```python
from build123d import *
from build123d.topology import SkipClean

# Parameters (mm, degrees)
EXTRUDE_1_DEPTH               = 15
CUT_EXTRUDE_1_DEPTH           = 4
SKETCH_3_R                    = 14
CUT_EXTRUDE_2_DEPTH           = 227.475164201
EXTRUDE_4_DEPTH               = 15
SKETCH_11_W                   = 17
SKETCH_11_H                   = 10
SKETCH_14_W                   = 6
SKETCH_14_H                   = 10
CUT_REVOLVE_4_ANGLE           = 60
CUT_REVOLVE_4_OTHER_WAY_ANGLE = 90
SKETCH_16_W                   = 9.609453317
SKETCH_16_H                   = 10
CUT_EXTRUDE_4_DEPTH           = 5
SKETCH_17_W                   = 9.609453317
SKETCH_17_H                   = 10
CUT_EXTRUDE_5_DEPTH           = 5
CUT_EXTRUDE_6_DEPTH           = 7.5
EXTRUDE_START                 = 1.5
EXTRUDE_6_DEPTH               = 1.5
SKETCH_21_R                   = 5
SKETCH_21_R_2                 = 14
EXTRUDE_7_DEPTH               = 1.5
HOLE_WIZARD_M4_1_D            = 3.3
HOLE_WIZARD_M4_1_DEPTH        = 9
HOLE_WIZARD_M4_1_CSINK_D      = 4.05
HOLE_WIZARD_M4_1_CSINK_ANGLE  = 90


with BuildPart() as part:
    # 草图1 → 凸台-拉伸1 (new body)
    with BuildSketch(Plane(origin=(0, 0, 0), x_dir=(1, 0, 0), z_dir=(0, 1, 0))):
        with BuildLine():
            Line((-21, 0), (-21, -215))
            ThreePointArc((-21, -215), (-18.071067812, -222.071067812), (-11, -225))
            Line((-11, -225), (-9.110127779, -225))
            ThreePointArc((-9.110127779, -225), (-2.375625019, -222.392325249), (0.846599179, -215.929294516))
            Line((0.846599179, -215.929294516), (21, 0))
            ThreePointArc((21, 0), (0, 21), (-21, 0))
        make_face()
    extrude(amount=EXTRUDE_1_DEPTH)

    # 草图2 → 切除-拉伸1 (cut)
    with BuildSketch(Plane.XZ):
        with BuildLine():
            Line((-6.487547308, 24.545681698), (-15.16946684, 197.954199749))
            ThreePointArc((-15.16946684, 197.954199749), (-9.006726896, 204.766554422), (-2.194372223, 198.603814478))
            Line((-2.194372223, 198.603814478), (6.487547308, 25.195296427))
            ThreePointArc((6.487547308, 25.195296427), (0.324807364, 18.382941754), (-6.487547308, 24.545681698))
        make_face()
    extrude(amount=-CUT_EXTRUDE_1_DEPTH, mode=Mode.SUBTRACT)

    # 草图3 → 切除-拉伸2 (cut, through all)
    with BuildSketch(Plane(origin=(0, 0, 0), x_dir=(-1, 0, 0), z_dir=(0, -1, 0))):
        with Locations(Location((0, 0, 0), (0, 0, 90))):
            Circle(SKETCH_3_R)
    extrude(amount=-CUT_EXTRUDE_2_DEPTH, mode=Mode.SUBTRACT)

    # 草图7 → 凸台-拉伸4 (add)
    with BuildSketch(Plane(origin=(0, 0, 0), x_dir=(1, 0, 0), z_dir=(0, 1, 0))):
        with BuildLine():
            Line((-10.693069191, 38.039100971), (-19.9158097, 6.66036966))
            ThreePointArc((-19.9158097, 6.66036966), (0, 21), (19.9158097, 6.66036966))
            Line((19.9158097, 6.66036966), (10.693069191, 38.039100971))
            ThreePointArc((10.693069191, 38.039100971), (0, 47.113526612), (-10.693069191, 38.039100971))
        make_face()
    extrude(amount=EXTRUDE_4_DEPTH)

    # 草图11 → 切除-旋转3 (revolve, cut)
    with BuildSketch(Plane(origin=(0, 0, 0), x_dir=(0, 0, -1), z_dir=(1, 0, 0)), mode=Mode.PRIVATE) as cut_revolve_3_sk:
        with Locations((51.539100971, 7.5)):
            Rectangle(SKETCH_11_W, SKETCH_11_H)
    revolve(cut_revolve_3_sk.sketch.rotate(Axis((0, 15, -38.039100971), (0, -1, 0)), 180), axis=Axis((0, 15, -38.039100971), (0, -1, 0)), mode=Mode.SUBTRACT)

    # 草图14 → 切除-旋转4 (revolve, cut)
    with BuildSketch(Plane(origin=(0, 0, 0), x_dir=(0, 0, -1), z_dir=(1, 0, 0))):
        with Locations((19.26034239, 7.5)):
            Rectangle(SKETCH_14_W, SKETCH_14_H)
    revolve(axis=Axis((0, 15, 0), (0, -1, 0)), revolution_arc=CUT_REVOLVE_4_ANGLE, mode=Mode.SUBTRACT)

    # 草图14 → 切除-旋转4 other way (revolve, cut)
    with BuildSketch(Plane(origin=(0, 0, 0), x_dir=(0, 0, -1), z_dir=(1, 0, 0))):
        with Locations((19.26034239, 7.5)):
            Rectangle(SKETCH_14_W, SKETCH_14_H)
    revolve(axis=Axis((0, 15, 0), (0, 1, 0)), revolution_arc=CUT_REVOLVE_4_OTHER_WAY_ANGLE, mode=Mode.SUBTRACT)

    # 草图16 → 切除-拉伸4 (cut)
    with BuildSketch(Plane(origin=(20.13407913, 0, -5.917746812), x_dir=(-0.2819890835944097, 0, -0.9594176133121516), z_dir=(0.9594176133121516, 0, -0.2819890835944097))):
        with Locations((12.229144047, 7.5)):
            Rectangle(SKETCH_16_W, SKETCH_16_H)
    extrude(amount=-CUT_EXTRUDE_4_DEPTH, mode=Mode.SUBTRACT)

    # 草图17 → 切除-拉伸5 (cut)
    with BuildSketch(Plane(origin=(-20.13407913, 0, -5.917746812), x_dir=(-0.28198908359441, 0, 0.9594176133121515), z_dir=(-0.9594176133121515, 0, -0.28198908359441))):
        with Locations((-12.229144047, 7.5)):
            Rectangle(SKETCH_17_W, SKETCH_17_H)
    extrude(amount=-CUT_EXTRUDE_5_DEPTH, mode=Mode.SUBTRACT)

    # 草图20 → 切除-拉伸6 (cut)
    with BuildSketch(Plane.XZ):
        with BuildLine():
            Line((21, 0), (0.846599179, 215.929294516))
            ThreePointArc((0.846599179, 215.929294516), (-2.375625019, 222.392325249), (-9.110127779, 225))
            Line((-9.110127779, 225), (-11, 225))
            ThreePointArc((-11, 225), (-18.071067812, 222.071067812), (-21, 215))
            Line((-21, 215), (-21, 0))
            ThreePointArc((-21, 0), (-20.727180268, -3.374018102), (-19.9158097, -6.66036966))
            Line((-19.9158097, -6.66036966), (-10.693069191, -38.039100971))
            ThreePointArc((-10.693069191, -38.039100971), (0, -47.113526612), (10.693069191, -38.039100971))
            Line((10.693069191, -38.039100971), (19.9158097, -6.66036966))
            ThreePointArc((19.9158097, -6.66036966), (20.727180268, -3.374018102), (21, 0))
        make_face()
    extrude(amount=-CUT_EXTRUDE_6_DEPTH, mode=Mode.SUBTRACT)

    # 草图22 → 凸台-拉伸6 (add)
    with BuildSketch(Plane.XZ.offset(-12.5).offset(EXTRUDE_START)):
        with BuildLine():
            Line((-19.9158097, -6.66036966), (-10.693069191, -38.039100971))
            ThreePointArc((-10.693069191, -38.039100971), (0, -47.113526612), (10.693069191, -38.039100971))
            Line((10.693069191, -38.039100971), (18.700124508, -10.796521919))
            Line((18.700124508, -10.796521919), (14.081869584, -8.130171195))
            ThreePointArc((14.081869584, -8.130171195), (8.995321483, -13.545586959), (2.030780118, -16.133030303))
            ThreePointArc((2.030780118, -16.133030303), (0, -16.039100971), (-2.030780118, -16.133030303))
            ThreePointArc((-2.030780118, -16.133030303), (-12.194669218, -10.755871759), (-16.26034239, 0))
            Line((-16.26034239, 0), (-21, 0))
            ThreePointArc((-21, 0), (-20.727180268, -3.374018102), (-19.9158097, -6.66036966))
        make_face()
    extrude(amount=-EXTRUDE_6_DEPTH)

    # 草图21 → 凸台-拉伸7 (add)
    # profile 1 of 2: a face of its own
    with SkipClean():  # the faces are left unmerged after this step: merging them gives an invalid solid
        with BuildSketch(Plane.XZ.offset(-7.5).offset(EXTRUDE_START)):
            with Locations(Location((0, -38.039100971, 0), (0, 0, 270))):
                Circle(SKETCH_21_R)
        # profile 2 of 2: a face of its own
        with BuildSketch(Plane.XZ.offset(-7.5).offset(EXTRUDE_START)):
            with BuildLine():
                Line((-21, 0), (-16.26034239, 0))
                ThreePointArc((-16.26034239, 0), (-12.194669218, -10.755871759), (-2.030780118, -16.133030303))
                ThreePointArc((-2.030780118, -16.133030303), (0, -16.039100971), (2.030780118, -16.133030303))
                ThreePointArc((2.030780118, -16.133030303), (8.995321483, -13.545586959), (14.081869584, -8.130171195))
                Line((14.081869584, -8.130171195), (18.700124508, -10.796521919))
                Line((18.700124508, -10.796521919), (19.9158097, -6.66036966))
                ThreePointArc((19.9158097, -6.66036966), (20.727180268, -3.374018102), (21, 0))
                Line((21, 0), (0.846599179, 215.929294516))
                ThreePointArc((0.846599179, 215.929294516), (-2.375625019, 222.392325249), (-9.110127779, 225))
                Line((-9.110127779, 225), (-11, 225))
                ThreePointArc((-11, 225), (-18.071067812, 222.071067812), (-21, 215))
                Line((-21, 215), (-21, 0))
            make_face()
            with Locations(Location((0, 0, 0), (0, 0, 270))):
                Circle(SKETCH_21_R_2, mode=Mode.SUBTRACT)
        extrude(amount=-EXTRUDE_7_DEPTH)

    # M4 螺纹孔1
    with Locations(Plane(origin=(0, 15, 0), x_dir=(1, 0, 0), z_dir=(0, 1, 0))):
        with Locations((-1.550565844, -196.226581502), (-4.338449392, -226.096762374), (-9.110127779, -215), (15.176735444, -17.005496271), (0, 38.039100971), (-15.5, -18.398087501), (-15.5, -48.398087501), (-15.5, -78.398087501), (-15.5, -108.398087501), (-15.5, -138.398087501), (-15.5, -168.398087501), (-15.5, -198.398087501), (12.388851896, -46.875677143), (9.600968348, -76.745858014), (6.8130848, -106.616038886), (4.025201252, -136.486219758), (1.237317704, -166.35640063)):
            CounterSinkHole(HOLE_WIZARD_M4_1_D / 2, HOLE_WIZARD_M4_1_CSINK_D / 2, depth=HOLE_WIZARD_M4_1_DEPTH, counter_sink_angle=HOLE_WIZARD_M4_1_CSINK_ANGLE)


solid = part.part
```
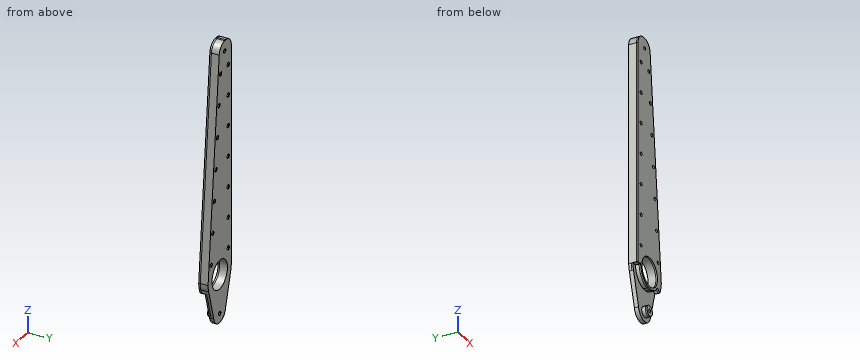
The listing builds one solid part. Answer for the finished solid, in the listing's coordinates (mm). Coordinates: 2 decimals unless noted, no trailing zeros. Loops run counter-clockwise (first coordinate to the right, second up) from the corner with the lowest first, then second, coordinate; pieces in that order, holes last. Notation, with made-up numbers: (12, -2.75) - (67, -2.75) arc R21 ccw to (67, 23.25) - close; hole circle Ø5 at (56, 72.5). An arc over 180 degrees is marked (long way). Write item = value, one per line.
1) Each of these flat-tipped pins is pushed along its axis until it touches: P1, Ø3, axis at x = -15.5, z = 108.4, coming from the -Y side; P2, Ø0.8, axis at x = -19, y = 6.5, coming from the -Z side; P3, Ø3, axis at x = -7.5, y = 8, coming from the -Z side; P4, Ø3, axis at x = 15, y = 8, coming from the -Z side. Where does it stop, or does it pass through?
Responses:
P1 = through
P2 = 0
P3 = -15.11
P4 = -9.53
2) Section B-B (z = 118) is taken. Determine the outline of the cut face in (x, y), plus the area to 3 significant figures.
Responses:
outline = (-21, 6) - (9.99, 6) - (9.99, 15) - (-21, 15) - close
area = 279 mm^2
3) Section A-A (z = 153.5) is taken. Determine the outline of the cut face in (x, y).
Responses:
outline = (-21, 6) - (6.67, 6) - (6.67, 15) - (-21, 15) - close
4) Find the intervals of material crossed by line 1 along Z through (x, y) = (-3, 10.5); line 2 along X through (y, z) = (13.5, 48); line 3 along Z through (x, y) = (-6, 14), in increasing order.
Responses:
line_1 = -42.04 to -34.04, -15.98 to -13.67, 13.67 to 195.44, 197.02 to 222.92
line_2 = -21 to -17.1, -13.9 to 11.18, 13.6 to 16.52
line_3 = -45.3 to -12.65, 12.65 to 224.5
